from build123d import *

# Parameters (mm, degrees)
SKETCH_1_W          = 56
SKETCH_1_H          = 30
SKETCH_1_R          = 2
EXTRUDE_1_DEPTH     = 3
SKETCH_2_W          = 41
SKETCH_2_H          = 4
EXTRUDE_2_DEPTH     = 26
SKETCH_3_W          = 62
SKETCH_3_H          = 40
EXTRUDE_3_DEPTH     = 3
CHAMFER_2_SIZE      = 3
CUT_EXTRUDE_1_DEPTH = 36
FILLET_1_R          = 2
CHAMFER_3_SIZE      = 3
CHAMFER_4_SIZE      = 3


with BuildPart() as part:
    # Эскиз1 → Бобышка-Вытянуть1 (new body)
    with BuildSketch(Plane(origin=(0, 0, 0), x_dir=(0, 0, -1), z_dir=(1, 0, 0))):
        with Locations((-20.5, 10.5)):
            Rectangle(SKETCH_1_W, SKETCH_1_H)
        with Locations((3.5, 15.5)):
            Circle(SKETCH_1_R, mode=Mode.SUBTRACT)
        with Locations((3.5, 5.5)):
            Circle(SKETCH_1_R, mode=Mode.SUBTRACT)
        with Locations((-44.5, 5.5)):
            Circle(SKETCH_1_R, mode=Mode.SUBTRACT)
        with Locations((-44.5, 15.5)):
            Circle(SKETCH_1_R, mode=Mode.SUBTRACT)
        with BuildLine():
            Line((0, 0), (-41, 0))
            Line((-41, 0), (-41, 21))
            Line((-41, 21), (0, 21))
            Line((0, 21), (0, 13.499943953))
            ThreePointArc((0, 13.499943953), (0.695596702, 13.218912412), (1, 12.533221423))
            Line((1, 12.533221423), (1, 8.663676138))
            ThreePointArc((1, 8.663676138), (0.771906654, 7.848193044), (0, 7.500056047))
            Line((0, 7.500056047), (0, 0))
        make_face(mode=Mode.SUBTRACT)
    extrude(amount=EXTRUDE_1_DEPTH)

    # Эскиз2 → Бобышка-Вытянуть2 (add)
    with BuildSketch(Plane.ZY):
        with Locations((20.5, 23.5)):
            Rectangle(SKETCH_2_W, SKETCH_2_H)
        with Locations((20.5, -2.5)):
            Rectangle(SKETCH_2_W, SKETCH_2_H)
    extrude(amount=EXTRUDE_2_DEPTH)

    # Эскиз3 → Бобышка-Вытянуть3 (add)
    with BuildSketch(Plane.ZY.offset(26)):
        with Locations((20.5, 10.5)):
            Rectangle(SKETCH_3_W, SKETCH_3_H)
    extrude(amount=EXTRUDE_3_DEPTH)

    # Фаска2
    chamfer_2_edges = [part.edges().sort_by_distance(p)[0] for p in [
        (-26, 25.5, 20.5),
        (-26, -4.5, 20.5),
    ]]
    chamfer(chamfer_2_edges, length=CHAMFER_2_SIZE)

    # Эскиз4 → Вырез-Вытянуть1 (cut, through all)
    with BuildSketch(Plane.XZ.offset(4.5)):
        with BuildLine():
            Line((-17, 33), (-9, 33))
            ThreePointArc((-9, 33), (-6.878679656, 32.121320344), (-6, 30))
            Line((-6, 30), (-6, 11))
            ThreePointArc((-6, 11), (-6.878679656, 8.878679656), (-9, 8))
            Line((-9, 8), (-17, 8))
            ThreePointArc((-17, 8), (-19.121320344, 8.878679656), (-20, 11))
            Line((-20, 11), (-20, 30))
            ThreePointArc((-20, 30), (-19.121320344, 32.121320344), (-17, 33))
        make_face()
    extrude(amount=-CUT_EXTRUDE_1_DEPTH, mode=Mode.SUBTRACT)

    # Скругление1
    fillet_1_edges = [part.edges().sort_by_distance(p)[0] for p in [
        (1.5, -4.5, -7.5),
        (1.5, -4.5, 48.5),
        (1.5, 25.5, 48.5),
        (1.5, 25.5, -7.5),
        (-27.5, 30.5, -10.5),
        (-27.5, -9.5, -10.5),
        (-27.5, -9.5, 51.5),
        (-27.5, 30.5, 51.5),
    ]]
    fillet(fillet_1_edges, radius=FILLET_1_R)

    # Фаска3
    chamfer_3_edges = [part.edges().sort_by_distance(p)[0] for p in [
        (0, 23.5, 0),
        (0, 23.5, 41),
        (0, -2.5, 0),
        (0, -2.5, 41),
    ]]
    chamfer(chamfer_3_edges, length=CHAMFER_3_SIZE)

    # Фаска4
    chamfer_4_edges = [part.edges().sort_by_distance(p)[0] for p in [
        (-26, 25, 0),
        (-26, -4, 0),
        (-26, 25, 41),
        (-26, -4, 41),
    ]]
    chamfer(chamfer_4_edges, length=CHAMFER_4_SIZE)


solid = part.part
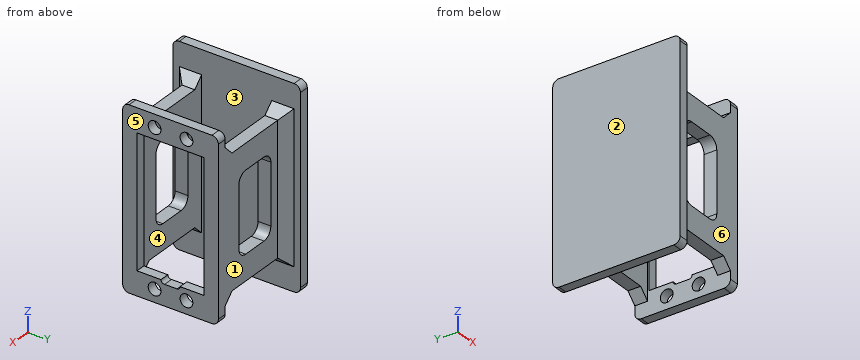
Could you check a few things on this model? Use its own coordinates, in mm. Face numbers are marked on the shaded views. A direction names the side the tool comes from. Give positions to 0.01 mm unless a question says otherwise; leave off trailing zeros. Order: outer loops, then holes, each group sorted by start corner. A loop starts at its lowest first (then second) coordinate and runs counter-clockwise, first axis right, second up. Notation, with made-up numbers: (54, 30.5) - (58, 30.5) arc R28 ccw to (58, 65.5) - close; hole circle Ø5 at (78.25, -7). An arc over 180 degrees is marked (long way). Return JSON: item names as keys, results as strings. Group by question number.
Q1. Suppose I cut it at D-D, the plane z = 16.5. Please give me the cut outline in (x, y), and give its area (3 significant figures).
Q2. Which directions (+Z, -Z, +X, -X, +Y, -Y) give clear straight access to the entire face, cutting with the end or side of a thin tool? Please do the marked faces 4, 5 and 6.
Q3. Suppose I cut it at B-B, the plane x = -10.5. Please give me the cut outline in (y, z), and give its area (3 significant figures).
Q4. Please list where these lines run through material, in increasing order: line 1 along Y through (x, z) = (-9.5, 6.5); line 2 along X through (y, z) = (-2.5, 44.5); line 3 along Y through (x, z) = (2.3, -3.5). Write a range as [from, to].
Q5. Will these pins go through, and if not, where does the flat tip stop? pin 1 Ø8 at (y, z) = (14.5, 22.5) entering from +X; pin 2 Ø6 at (x, y) = (-11.5, 17) entering from +Z; pin 3 Ø4.5 at (x, y) = (-13, 24) entering from -Z; pin 4 Ø1.5 at (x, y) = (1, 11) entering from +Z.
Q6. Thinking about a two-plate mould opening in Y: for the marked faces 1, 2 and 3, which applies, pulls with the +Y half, pulls with the -Y half, needs draft (parallel to the pull), parting line crosses it, or undercut?
Q7. Suppose I cut it at A-A, the plane y = 5.5. Please give me the cut outline in (x, z), and give its area (3 significant figures).
Q8. Suppose I cut it at C-C, the plane y = 1.5. Please give me the cut outline in (x, z).
Resolved:
{
 "1": {"outline": "(-29, -9.5) - (-26, -9.5) - (-26, -7.5) - (-23, -4.5) - (-20, -4.5) - (-20, -0.5) - (-26, -0.5) - (-26, 21.5) - (-20, 21.5) - (-20, 25.5) - (-23, 25.5) - (-26, 28.5) - (-26, 30.5) - (-29, 30.5) - close; (-6, -4.5) - (3, -4.5) - (3, 0) - (0, 0) - (0, -0.5) - (-6, -0.5) - close; (-6, 21.5) - (0, 21.5) - (0, 21) - (3, 21) - (3, 25.5) - (-6, 25.5) - close", "area": "252 mm2"},
 "2": {"face 4": "+Z, -Z", "face 5": "+Z, -Z, +X, +Y, -Y", "face 6": "+Z, -Z, +X, -Y"},
 "3": {"outline": "(-4.5, 0) - (-0.5, 0) - (-0.5, 8) - (-4.5, 8) - close; (-4.5, 33) - (-0.5, 33) - (-0.5, 41) - (-4.5, 41) - close; (21.5, 0) - (25.5, 0) - (25.5, 8) - (21.5, 8) - close; (21.5, 33) - (25.5, 33) - (25.5, 41) - (21.5, 41) - close", "area": "128 mm2"},
 "4": {"line 1": "y = [-4.5, -0.5], [21.5, 25.5]", "line 2": "x = [-29, -26], [0, 3]", "line 3": "y = [-4.5, 3.5], [7.5, 13.5], [17.5, 25.5]"},
 "5": {"pin 1": "stops at x = -26", "pin 2": "passes through", "pin 3": "stops at z = 0", "pin 4": "stops at z = 48.5"},
 "6": {"face 1": "pulls with the +Y half", "face 2": "needs draft", "face 3": "undercut"},
 "7": {"outline": "(-29, -10.5) - (-26, -10.5) - (-26, 51.5) - (-29, 51.5) - close; (0, -7.5) - (3, -7.5) - (3, -5.5) - (0, -5.5) - close; (0, -1.5) - (3, -1.5) - (3, 0) - (0, 0) - close; (0, 41) - (3, 41) - (3, 42.5) - (0, 42.5) - close; (0, 46.5) - (3, 46.5) - (3, 48.5) - (0, 48.5) - close", "area": "207 mm2"},
 "8": {"outline": "(-29, -10.5) - (-26, -10.5) - (-26, 51.5) - (-29, 51.5) - close; (0, -7.5) - (3, -7.5) - (3, 0) - (0, 0) - close; (0, 41) - (3, 41) - (3, 48.5) - (0, 48.5) - close"}
}
